```python
from build123d import *

# Parameters (mm, degrees)
F0_R     = 25
F1_DEPTH = 4
F3_DEPTH = 5


with BuildPart() as f1:
    # F0 (on Top) → F1 (new body)
    with BuildSketch(Plane.XY):
        Circle(F0_R)
    extrude(amount=F1_DEPTH)

    # F2 (on face) → F3 (cut)
    with BuildSketch(Plane.XY.offset(4)):
        with BuildLine():
            Line((-17.318032, 10.358936), (-17.318032, 13.241064))
            ThreePointArc((-17.318032, 13.241064), (-21.8, 0), (-17.318032, -13.241064))
            Line((-17.318032, -13.241064), (-17.318032, -5.958936))
            Line((-17.318032, -5.958936), (-17.318032, -2.958936))
            Line((-17.318032, -2.958936), (-10.118032, -2.958936))
            Line((-10.118032, -2.958936), (-10.118032, -5.958936))
            Line((-10.118032, -5.958936), (-10.118032, -10.358936))
            Line((-10.118032, -10.358936), (-8.518032, -10.358936))
            ThreePointArc((-8.518032, -10.358936), (-6.718569, -9.835054), (-5.040088, -9.001257))
            ThreePointArc((-5.040088, -9.001257), (-6.874725, -4.658377), (-7.6, 0))
            ThreePointArc((-7.6, 0), (-6.874725, 4.658377), (-5.040088, 9.001257))
            ThreePointArc((-5.040088, 9.001257), (-6.718569, 9.835054), (-8.518032, 10.358936))
            Line((-8.518032, 10.358936), (-10.118032, 10.358936))
            Line((-10.118032, 10.358936), (-10.118032, 3.041064))
            Line((-10.118032, 3.041064), (-17.318032, 3.041064))
            Line((-17.318032, 3.041064), (-17.318032, 10.358936))
        make_face()
        with BuildLine():
            ThreePointArc((0, 0), (-0.253032, 2.297592), (-1, 4.485056))
            ThreePointArc((-1, 4.485056), (-1.746968, 2.297592), (-2, 0))
            ThreePointArc((-2, 0), (-1.746968, -2.297592), (-1, -4.485056))
            ThreePointArc((-1, -4.485056), (-0.253032, -2.297592), (0, 0))
        make_face()
        with BuildLine():
            Line((6.518032, 17.958936), (12.357857, 17.958936))
            ThreePointArc((12.357857, 17.958936), (0, 21.8), (-12.357857, 17.958936))
            Line((-12.357857, 17.958936), (-8.518032, 17.958936))
            ThreePointArc((-8.518032, 17.958936), (-4.532276, 16.358457), (-1, 13.914934))
            ThreePointArc((-1, 13.914934), (2.532276, 16.358457), (6.518032, 17.958936))
        make_face()
        with BuildLine():
            ThreePointArc((15.318032, -15.511219), (20.114337, -8.405561), (21.8, 0))
            ThreePointArc((21.8, 0), (20.114337, 8.405561), (15.318032, 15.511219))
            Line((15.318032, 15.511219), (15.318032, 10.358936))
            Line((15.318032, 10.358936), (15.318032, 5))
            Line((15.318032, 5), (8.118032, 5))
            Line((8.118032, 5), (8.118032, 10.358936))
            Line((8.118032, 10.358936), (6.518032, 10.358936))
            ThreePointArc((6.518032, 10.358936), (4.718569, 9.835054), (3.040088, 9.001257))
            ThreePointArc((3.040088, 9.001257), (4.874725, 4.658377), (5.6, 0))
            ThreePointArc((5.6, 0), (4.874725, -4.658377), (3.040088, -9.001257))
            ThreePointArc((3.040088, -9.001257), (4.718569, -9.835054), (6.518032, -10.358936))
            Line((6.518032, -10.358936), (8.118032, -10.358936))
            Line((8.118032, -10.358936), (8.118032, -4.999936))
            Line((8.118032, -4.999936), (15.318032, -4.999936))
            Line((15.318032, -4.999936), (15.318032, -10.358936))
            Line((15.318032, -10.358936), (15.318032, -15.511219))
        make_face()
        with BuildLine():
            ThreePointArc((-12.357857, -17.958936), (0, -21.8), (12.357857, -17.958936))
            Line((12.357857, -17.958936), (10.357857, -17.958936))
            Line((10.357857, -17.958936), (6.518032, -17.958936))
            ThreePointArc((6.518032, -17.958936), (2.532276, -16.358457), (-1, -13.914934))
            ThreePointArc((-1, -13.914934), (-4.532276, -16.358457), (-8.518032, -17.958936))
            Line((-8.518032, -17.958936), (-12.357857, -17.958936))
        make_face()
    extrude(amount=-F3_DEPTH, mode=Mode.SUBTRACT)


solid = f1.part
```
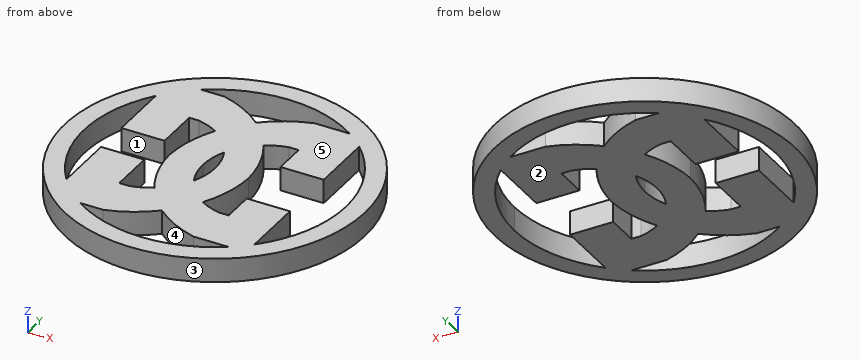
Could you check a few things on this model? Use its own coordinates, in mm. Face numbers are marked on the shaded views. A direction names the side the tool comes from. Coordinates: 2 decimals unless noted, no trailing zeros. Write each loop counter-clockwise with the first axis right and the second up, starting at its lowest first coordinate (ties: lowest second). Pieces come first, ordered by that corner, then holes. Notation, with made-up numbers: (-26.5, 80.5) -> (2.5, 80.5) arc R27 ccw to (2.5, 96.5) -> close; hole circle Ø3 at (75.5, 17.25). An arc over 180 degrees is marked (long way). Write item = value, one per line. Start each with the question number.
(1) I want a section at D-D (x = 20.5). Please give me the cut outline in (y, z).
(2) I need wall thicknesses on line 1 (Y direction, x = -11, z = 1.6); line 2 (Y direction, x = -9, z = 0.75); line 3 (X direction, y = -12, z = 0.55). Which ranges of each line are inside material? Lowest first, please. Write a range as [from, to].
(3) I want a section at C-C (z = 1.4). Give the number of separate pieces and of enclosed holes in the cut face, plus the area to 3 significant figures.
(4) I want a section at A-A (x = -16.5). Please give me the cut outline in (y, z), plus the area to 3 significant figures.
(5) Which directions (+Z, -Z, +X, -X, +Y, -Y) give clear straight access to the entire face, cutting with the end or side of a thin tool? Please do the marked faces 4 and 5.
(6) I want a section at B-B (x = -3). Please give me the cut outline in (y, z), plus the area to 3 significant figures.
(7) Will these pins go through, and if not, where does the flat tip stop? pin 1 (2 mm diameter, centred on y = -11.5, z = 2.5, fed in from +X); pin 2 (2 mm diameter, centred on x = 17.5, z = 2.5, fed in from -Y); pin 3 (1.9 mm diameter, centred on x = -10, z = 1, fed in from +Y).
(8) We'd pull the mould along Y, two halves only. Please class the marked faces 1, 2 and 3: released by +Y, released by -Y, zero draft, split by the parting line, or undercut.
Result set:
q1.outline = (-14.31, 0) -> (-7.42, 0) -> (-7.42, 4) -> (-14.31, 4) -> close; (7.42, 0) -> (14.31, 0) -> (14.31, 4) -> (7.42, 4) -> close
q2.line_1 = [-22.45, -18.82], [-17.96, -2.96], [3.04, 17.96], [18.82, 22.45]
q2.line_2 = [-23.32, -19.86], [-17.96, -10.36], [10.36, 17.96], [19.86, 23.32]
q2.line_3 = [-21.93, -18.2], [-17.32, 15.32], [18.2, 21.93]
q3.separate_pieces = 1
q3.enclosed_holes = 5
q3.area = 1,300 mm2
q4.outline = (-18.78, 0) -> (-2.96, 0) -> (-2.96, 4) -> (-18.78, 4) -> close; (3.04, 0) -> (18.78, 0) -> (18.78, 4) -> (3.04, 4) -> close
q4.area = 126 mm2
q5.face_4 = +Z, -Z
q5.face_5 = +Z, +X, -X, +Y, -Y
q6.outline = (-24.82, 0) -> (-21.59, 0) -> (-21.59, 4) -> (-24.82, 4) -> close; (-15.44, 0) -> (15.44, 0) -> (15.44, 4) -> (-15.44, 4) -> close; (21.59, 0) -> (24.82, 0) -> (24.82, 4) -> (21.59, 4) -> close
q6.area = 149 mm2
q7.pin_1 = 22.69
q7.pin_2 = -18.78
q7.pin_3 = 23.3
q8.face_1 = undercut
q8.face_2 = zero draft
q8.face_3 = split by the parting line
